```python
from build123d import *

# Parameters (mm, degrees)
F0_W     = 17.8
F0_H     = 16
F1_DEPTH = 5
F2_R     = 1.7
F3_DEPTH = 5.001


with BuildPart() as f1:
    # F0 (on Front) → F1 (new body)
    with BuildSketch(Plane.XZ):
        with Locations((8.9, -8)):
            Rectangle(F0_W, F0_H)
    extrude(amount=-F1_DEPTH)

    # F2 (on face) → F3 (cut, through all)
    with BuildSketch(Plane.XZ):
        with Locations((3.2, -11.6)):
            Circle(F2_R)
        with Locations((14.6, -4.4)):
            Circle(F2_R)
    extrude(amount=-F3_DEPTH, mode=Mode.SUBTRACT)


solid = f1.part
```
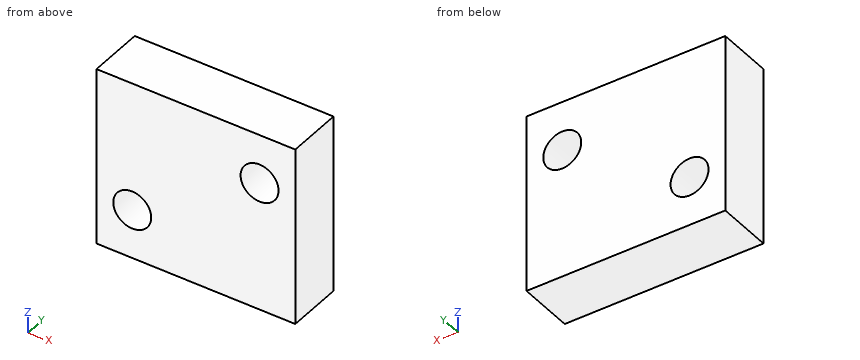
Can you work these out from the model? Positions are in its coordinate system, mm. Coordinates: 2 decimals unless noted, no trailing zeros. Order: outer loops, then holes, each group sorted by start corner. A loop starts at its lowest first (then second) coordinate and runs counter-clockwise, first axis right, second up. Notation, with made-up numbers: (72.5, 24.25) - (123.5, 24.25) arc R35 cw to (123.5, 59.25) - close; hole circle Ø6 at (9.25, 2). An arc over 180 degrees is marked (long way). Answer in a Markdown table with one row per item.
1. Suppose I cut it at B-B (z = -10.75). Please give me the cut outline in (x, y).
Reply:
| item | result |
|---|---|
| outline | (0, 0) - (1.73, 0) - (1.73, 5) - (0, 5) - close; (4.67, 0) - (17.8, 0) - (17.8, 5) - (4.67, 5) - close |
2. Suppose I cut it at A-A (x = 3.2). Please give me the cut outline in (y, z).
Reply:
| item | result |
|---|---|
| outline | (0, -16) - (5, -16) - (5, -13.3) - (0, -13.3) - close; (0, -9.9) - (5, -9.9) - (5, 0) - (0, 0) - close |
3. For pin 1 (2.5 mm diameter, centred on x = 3.2, z = -11.6, fed in from -Y), with a flat end and sliding along its axis, tell me the tip position at first contact or that it passes through.
Reply:
| item | result |
|---|---|
| pin 1 | passes through |
4. If I drill on line 1 along Z through (x, y) = (3.2, 3.05); line 2 along Z through (x, y) = (14.6, 2.6); line 3 along X through (y, z) = (1.9, -11.5), over which ranges is the centre line in solid material (lowest first)?
Reply:
| item | result |
|---|---|
| line 1 | z = -16 to -13.3, -9.9 to 0 |
| line 2 | z = -16 to -6.1, -2.7 to 0 |
| line 3 | x = 0 to 1.5, 4.9 to 17.8 |
5. Suppose I cut it at C-C (y = 1.9). Please give me the cut outline in (x, z).
Reply:
| item | result |
|---|---|
| outline | (0, -16) - (17.8, -16) - (17.8, 0) - (0, 0) - close; hole circle Ø3.4 at (3.2, -11.6); hole circle Ø3.4 at (14.6, -4.4) |
